Verification items for the finished model (mm, model axes). Face numbers are marked on the shaded views. A direction names the side the tool comes from. Coordinates: 2 decimals unless noted, no trailing zeros. Loops run counter-clockwise (first coordinate to the right, second up) from the corner with the lowest first, then second, coordinate; pieces in that order, holes last.
Q1. Material ranges on probe 1 along Z at (x, y) = (-7.75, 14.5); probe 2 along Z at (x, y) = (2.5, 9); probe 3 along X at (y, z) = (-2, -23), recorded low to high.
Q2. Access from +Z, -Z, +X, -X, +Y, -Y to the whole of each face (thin tool, end or side, straight path). Record for the marked faces 1, 2 and 3.
Q3. Sectioned sample at B-B (y = 11.5). Enter the section's corners in (x, z).
Q4. Go/stop test with flat-tipped pins: P1, Ø3, axis at x = -1, z = -4, coming from the -Y side; P2, Ø0.7, axis at y = 3, z = -17, coming from the -X side; P3, Ø8, axis at y = 3, z = -23, coming from the +X side. Record where each tip stops, or that it passes through.
Q5. Sectioned sample at D-D (z = -2). Enter the section's corners in (x, y).
Q6. Mould release check, pull along X, two halves, no side actions. Record for the marked faces 4, 5 and 6: +X half, -X half, draft (parallel to the pull), parting line (faces both ways), or undercut.
Q7. Sectioned sample at A-A (z = -15). Enter the section's corners in (x, y) (3 decimals), then the cut area to 3 significant figures.
Q8. Sectioned sample at C-C (z = 3). Enter the section's corners in (x, y), then the cut area to 3 significant figures.
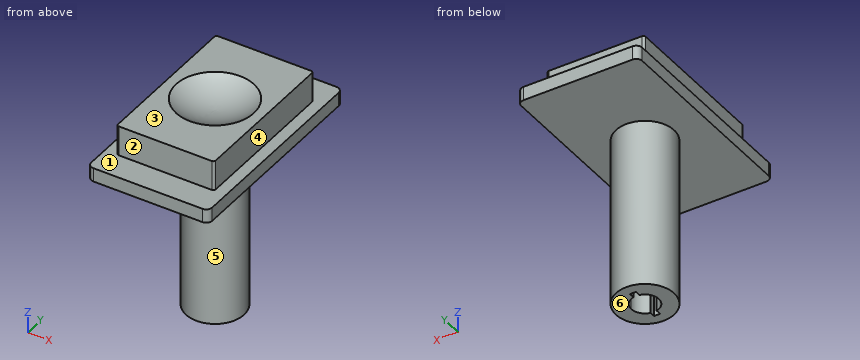
```python
from build123d import *

# Parameters (mm, degrees)
SKETCH1_W           = 35
SKETCH1_H           = 20.2
BOSS_EXTRUDE1_DEPTH = 2.3
SKETCH2_W           = 16.3
SKETCH2_H           = 25.9
BOSS_EXTRUDE2_DEPTH = 5
FILLET2_R           = 1
FILLET3_R           = 0.4
SKETCH5_R           = 4.85
BOSS_EXTRUDE3_DEPTH = 28.2
CUT_EXTRUDE3_DEPTH  = 16


with BuildPart() as part:
    # Sketch1 → Boss-Extrude1 (new body)
    with BuildSketch(Plane(origin=(0, 0, 0), x_dir=(0, 1, 0), z_dir=(0, 0, 1))):
        Rectangle(SKETCH1_W, SKETCH1_H)
    extrude(amount=BOSS_EXTRUDE1_DEPTH)

    # Sketch2 → Boss-Extrude2 (add)
    with BuildSketch(Plane.XY.offset(2.3)):
        Rectangle(SKETCH2_W, SKETCH2_H)
    extrude(amount=BOSS_EXTRUDE2_DEPTH)

    # Sketch4 → Cut-Revolve1 (revolve, cut)
    with BuildSketch(Plane.YZ):
        with BuildLine():
            Line((0, 7.3), (-6.5, 7.3))
            ThreePointArc((-6.5, 7.3), (-3.398426688, 5.817613265), (0, 5.3))
            Line((0, 5.3), (0, 7.3))
        make_face()
    revolve(axis=Axis((0, 0, 0), (0, 0, 1)), mode=Mode.SUBTRACT)

    # Fillet2
    fillet2_edges = [part.edges().sort_by_distance(p)[0] for p in [
        (10.1, 17.5, 1.15),
        (10.1, -17.5, 1.15),
        (-10.1, -17.5, 1.15),
        (-10.1, 17.5, 1.15),
    ]]
    fillet(fillet2_edges, radius=FILLET2_R)

    # Fillet3
    fillet3_edges = [part.edges().sort_by_distance(p)[0] for p in [
        (8.15, -12.95, 4.8),
        (8.15, 12.95, 4.8),
        (-8.15, 12.95, 4.8),
        (-8.15, -12.95, 4.8),
    ]]
    fillet(fillet3_edges, radius=FILLET3_R)

    # Sketch5 → Boss-Extrude3 (add)
    with BuildSketch(Plane(origin=(0, 0, 0), x_dir=(1, 0, 0), z_dir=(0, 0, -1))):
        Circle(SKETCH5_R)
    extrude(amount=BOSS_EXTRUDE3_DEPTH)

    # Sketch6 → Cut-Extrude3 (cut)
    with BuildSketch(Plane(origin=(0, 0, -28.2), x_dir=(1, 0, 0), z_dir=(0, 0, -1))):
        with BuildLine():
            Line((-0.5, 3.15), (-0.5, 2.244994432))
            ThreePointArc((-0.5, 2.244994432), (0, 2.3), (0.5, 2.244994432))
            Line((0.5, 2.244994432), (0.5, 3.15))
            Line((0.5, 3.15), (-0.5, 3.15))
        make_face()
        with BuildLine():
            Line((0.5, 1.45), (-0.5, 1.45))
            Line((-0.5, 1.45), (-0.5, 2.244994432))
            ThreePointArc((-0.5, 2.244994432), (-2.3, 0), (-0.5, -2.244994432))
            Line((-0.5, -2.244994432), (-0.5, -1.45))
            Line((-0.5, -1.45), (0.5, -1.45))
            Line((0.5, -1.45), (0.5, -2.244994432))
            ThreePointArc((0.5, -2.244994432), (1.794435844, -1.438749457), (2.3, 0))
            ThreePointArc((2.3, 0), (1.794435844, 1.438749457), (0.5, 2.244994432))
            Line((0.5, 2.244994432), (0.5, 1.45))
        make_face()
        with BuildLine():
            ThreePointArc((0.5, -2.244994432), (0, -2.3), (-0.5, -2.244994432))
            Line((-0.5, -2.244994432), (-0.5, -3.15))
            Line((-0.5, -3.15), (0.5, -3.15))
            Line((0.5, -3.15), (0.5, -2.244994432))
        make_face()
        with BuildLine():
            Line((-0.5, 2.244994432), (-0.5, 1.45))
            Line((-0.5, 1.45), (0.5, 1.45))
            Line((0.5, 1.45), (0.5, 2.244994432))
            ThreePointArc((0.5, 2.244994432), (0, 2.3), (-0.5, 2.244994432))
        make_face()
        with BuildLine():
            Line((-0.5, -1.45), (-0.5, -2.244994432))
            ThreePointArc((-0.5, -2.244994432), (0, -2.3), (0.5, -2.244994432))
            Line((0.5, -2.244994432), (0.5, -1.45))
            Line((0.5, -1.45), (-0.5, -1.45))
        make_face()
    extrude(amount=-CUT_EXTRUDE3_DEPTH, mode=Mode.SUBTRACT)


solid = part.part
```
Geometry check:
1. probe 1: z = 0 to 2.3
1. probe 2: z = 0 to 7.3
1. probe 3: x = -4.42 to -1.14, 1.14 to 4.42
2. face 1: +Z
2. face 2: +Z, +X, -X, -Y
2. face 3: +Z, +X, -X, +Y, -Y
3. outline: (-10.1, 0) - (10.1, 0) - (10.1, 2.3) - (8.15, 2.3) - (8.15, 7.3) - (-8.15, 7.3) - (-8.15, 2.3) - (-10.1, 2.3) - close
4. P1: stops at y = -4.85
4. P2: stops at x = -4.06
4. P3: stops at x = 4.85
5. outline: circle Ø9.7 at (0, 0)
6. face 4: +X half
6. face 5: parting line
6. face 6: draft
7. outline: circle Ø9.7 at (0, 0); hole (-0.5, -3.15) - (0.5, -3.15) - (0.5, -2.245) arc R2.3 ccw to (0.5, 2.245) - (0.5, 3.15) - (-0.5, 3.15) - (-0.5, 2.245) arc R2.3 ccw to (-0.5, -2.245) - close
7. area: 55.5 mm2
8. outline: (-8.15, -12.55) arc R0.4 ccw to (-7.75, -12.95) - (7.75, -12.95) arc R0.4 ccw to (8.15, -12.55) - (8.15, 12.55) arc R0.4 ccw to (7.75, 12.95) - (-7.75, 12.95) arc R0.4 ccw to (-8.15, 12.55) - close
8. area: 422 mm2
